The listing builds one solid part. Answer for the finished solid, in the listing's coordinates (mm). A direction names the side the tool comes from. Coordinates: 2 decimals unless noted, no trailing zeros. Order: outer loops, then holes, each group sorted by start corner. A loop starts at its lowest first (then second) coordinate and runs counter-clockwise, first axis right, second up. Notation, with made-up numbers: (17, -24) -> (27, -24) arc R21 cw to (27, -11) -> close; hole circle Ø9 at (31, 20). An arc over 180 degrees is marked (long way). Write item = value, one per line.
from build123d import *

# Parameters (mm, degrees)
F1_DEPTH = 68.326
F2_W     = 87.6199703779
F2_H     = 65.060084963
F2_W_2   = 70.4743001366
F2_H_2   = 87.6017467856
F3_DEPTH = 140.2725
F9_DEPTH = 19.05


with BuildPart() as f1:
    # F0 (on Front) → F1 (new body)
    with BuildSketch(Plane.XZ):
        with BuildLine():
            Line((-140.2715, 0), (0, 0))
            Line((0, 0), (0, 28.575))
            Line((0, 28.575), (-104.1369961518, 77.1348788028))
            ThreePointArc((-104.1369961518, 77.1348788028), (-128.518910052, 75.5368037358), (-140.2715, 54.1146610121))
            Line((-140.2715, 54.1146610121), (-140.2715, 0))
        make_face()
    extrude(amount=F1_DEPTH)

    # F2 (on Right) → F3 (cut, through all)
    with BuildSketch(Plane.YZ):
        with Locations((-82.925985189, -18.1790424815)):
            Rectangle(F2_W, F2_H)
        with Locations((-83.4971500683, 72.3758733928)):
            Rectangle(F2_W_2, F2_H_2)
    extrude(amount=-F3_DEPTH, mode=Mode.SUBTRACT)

    # F5 (on offset) → F6 (revolve, cut)
    with BuildSketch(Plane(origin=(0, -22.225, 0), x_dir=(-1, 0, 0), z_dir=(0, 1, 0))):
        Polygon((71.1155433788, 30.3478274527), (50.8693131181, 73.7660083611), (39.2441031338, 68.3450839177), (62.7475534112, 17.9417721419), align=None)
    revolve(axis=Axis((-50.9958282725, -22.225, 43.1434280298), (-0.4226182617, 0, -0.906307787)), mode=Mode.SUBTRACT)

    # F8 (on offset) → F9 (cut)
    with BuildSketch(Plane(origin=(0, -15.748, 0), x_dir=(-1, 0, 0), z_dir=(0, 1, 0))):
        Polygon((164.5451933146, 38.0492), (164.5451933146, 123.7454637885), (43.1606759201, 123.7454637885), (83.1215, 38.0492), align=None)
    extrude(amount=-F9_DEPTH, mode=Mode.SUBTRACT)


solid = f1.part
Q1. The mould has two halves that part along Z. Classify faces 6 (the face through (-50.875, -34.747, 36.824)), 7 (the face through (-39.77, -34.52, 47.12)), 8 (the face through (-69, -54, 14.351)): released by +Z, released by -Z, zero draft, split by the parting line, or undercut.
The answers:
face_6 = undercut
face_7 = released by +Z
face_8 = released by -Z
Q2. Section A-A, the plane y = -46 is taken. Give the vertices of the cut face in (x, z) (1 decimal), plus the area to 3 significant figures.
The answers:
outline = (-140.3, 14.4) -> (0, 14.4) -> (0, 28.6) -> (-104.1, 77.1) arc R25.4 ccw to (-140.3, 54.1) -> close
area = 6,220 mm2
Q3. Section C-C, the plane x = -81 is taken. Give the vertices of the cut face in (y, z) (3 decimals).
The answers:
outline = (-68.326, 14.351) -> (-39.116, 14.351) -> (-39.116, 0) -> (0, 0) -> (0, 66.346) -> (-15.748, 66.346) -> (-15.748, 42.599) -> (-34.798, 42.599) -> (-34.798, 66.346) -> (-48.26, 66.346) -> (-48.26, 28.575) -> (-68.326, 28.575) -> close
Q4. Each of these flat-tipped pins is pushed along its axis until it touches: pin 1 Ø4 at (x, y) = (-122, -49.5) entering from -Z; pin 2 Ø12 at (x, z) = (-121.5, 9.5) entering from +Y; pin 3 Ø3 at (x, z) = (-67.5, 48) entering from -Y; pin 4 Ø1.5 at (x, y) = (-105.5, -8.5) entering from +Z. Where does it stop, or does it pass through?
The answers:
pin_1 = 14.35
pin_2 = 0
pin_3 = -48.26
pin_4 = 78.01
Q5. Section B-B, the plane z = 5.5 is taken. Give the vertices of the cut face in (x, y), plus the area to 3 significant figures.
The answers:
outline = (-140.27, -39.12) -> (0, -39.12) -> (0, 0) -> (-140.27, 0) -> close
area = 5,490 mm2
Q6. Section D-D, the plane y = -6.5 is taken. Give the vertices of the cut face in (x, z) (1 decimal), plus the area to 3 significant figures.
The answers:
outline = (-140.3, 0) -> (0, 0) -> (0, 28.6) -> (-104.1, 77.1) arc R25.4 ccw to (-140.3, 54.1) -> close
area = 8,230 mm2
Q7. A tool of negligible diameter and unlimited length cuts with its end or side. For faces 1 (the face through (-69, -39.116, 7)), 2 (the face through (-85, -48.26, 48)), 3 (the face through (-140.272, -26, 21)), 4 (the face through (-60.165, -22.127, 18.214)), 5 (the face through (-111, -25, 38.049)), from which of +Z, -Z, +X, -X, +Y, -Y can it reach the whole face along a straight path? Write none if from no direction.
The answers:
face_1 = -Z, +X, -X, -Y
face_2 = +Z, +X, -X, -Y
face_3 = +Z, -Z, -X, +Y, -Y
face_4 = none
face_5 = +Z, -X
Q8. Find the intervals of material crossed by line 1 along Y through (x, z) = (-91.5, 48.5); line 2 along Z through (x, y) = (-24.5, -50.5) (3 decimals); line 3 along X through (y, z) = (-13.5, 26), in increasing order.
The answers:
line_1 = -48.26 to -34.8, -15.75 to 0
line_2 = 14.351 to 28.575
line_3 = -140.27 to -65.24, -48.62 to 0
